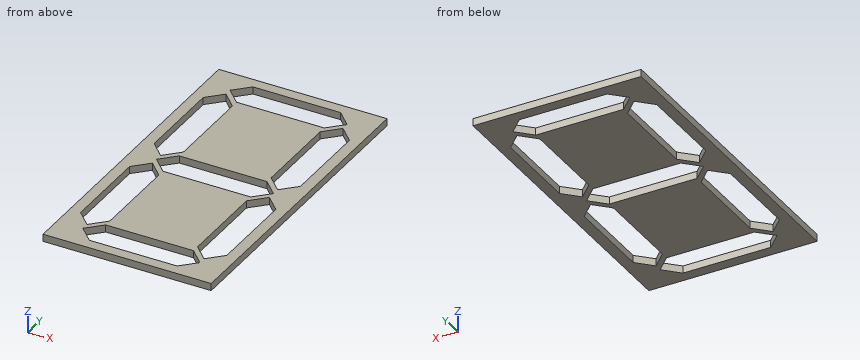
```python
from build123d import *

# Parameters (mm, degrees)
BOX011_W         = 46
BOX011_H         = 4
BOX011_DEPTH     = 10
BOX010_W         = 1
BOX010_H         = 90
BOX010_DEPTH     = 2
BOX_W            = 1
BOX_H            = 90
BOX_DEPTH        = 2
EXTRUDE006_DEPTH = 10
EXTRUDE005_DEPTH = 10
EXTRUDE004_DEPTH = 10
EXTRUDE_DEPTH    = 10
EXTRUDE003_DEPTH = 10
EXTRUDE002_DEPTH = 10
EXTRUDE001_DEPTH = 10
BOX001_W         = 44
BOX001_H         = 90
BOX001_DEPTH     = 2


with BuildPart() as cube011:
    # Box011 → Box011 (new body)
    with BuildSketch(Plane(origin=(-1, 86, -4), x_dir=(1, 0, 0), z_dir=(0, 0, 1))):
        with Locations((23, 2)):
            Rectangle(BOX011_W, BOX011_H)
    extrude(amount=BOX011_DEPTH)


with BuildPart() as cube010:
    # Box010 → Box010 (new body)
    with BuildSketch(Plane(origin=(44, 0, 0), x_dir=(1, 0, 0), z_dir=(0, 0, 1))):
        with Locations((0.5, 45)):
            Rectangle(BOX010_W, BOX010_H)
    extrude(amount=BOX010_DEPTH)


with BuildPart() as cube:
    # Box → Box (new body)
    with BuildSketch(Plane(origin=(-1, 0, 0), x_dir=(1, 0, 0), z_dir=(0, 0, 1))):
        with Locations((0.5, 45)):
            Rectangle(BOX_W, BOX_H)
    extrude(amount=BOX_DEPTH)


with BuildPart() as extrude_g:
    # Sketch008 (on Face6 of Box006) → Extrude006 (new body)
    with BuildSketch(Plane.XY.offset(10)):
        Polygon((10, 47), (6, 43), (10, 39), (34, 39), (38, 43), (34, 47), align=None)
    extrude(amount=EXTRUDE006_DEPTH)


with BuildPart() as extrude_g_1:
    # Extrude006 placement: moved
    add(extrude_g.part.moved(Location((0, 0, -14))))


with BuildPart() as extrude_f:
    # Sketch010 (on Face6 of Box008) → Extrude005 (new body)
    with BuildSketch(Plane.XY.offset(10)):
        Polygon((6, 77), (10, 73), (10, 49), (6, 45), (2, 49), (2, 73), align=None)
    extrude(amount=EXTRUDE005_DEPTH)


with BuildPart() as extrude_f_1:
    # Extrude005 placement: moved
    add(extrude_f.part.moved(Location((0, 0, -14))))


with BuildPart() as extrude_e:
    # Sketch011 (on Face6 of Box009) → Extrude004 (new body)
    with BuildSketch(Plane.XY.offset(10)):
        Polygon((6, 41), (10, 37), (10, 13), (6, 9), (2, 13), (2, 37), align=None)
    extrude(amount=EXTRUDE004_DEPTH)


with BuildPart() as extrude_e_1:
    # Extrude004 placement: moved
    add(extrude_e.part.moved(Location((0, 0, -14))))


with BuildPart() as extrude_d:
    # Sketch003 (on Face6 of Box001) → Extrude (new body)
    with BuildSketch(Plane.XY.offset(2)):
        Polygon((10, 11), (6, 7), (10, 3), (34, 3), (38, 7), (34, 11), align=None)
    extrude(amount=EXTRUDE_DEPTH)


with BuildPart() as extrude_d_1:
    # Extrude placement: moved
    add(extrude_d.part.moved(Location((0, 0, -6))))


with BuildPart() as extrude_c:
    # Sketch006 (on Face6 of Box004) → Extrude003 (new body)
    with BuildSketch(Plane.XY.offset(10)):
        Polygon((38, 41), (42, 37), (42, 13), (38, 9), (34, 13), (34, 37), align=None)
    extrude(amount=EXTRUDE003_DEPTH)


with BuildPart() as extrude_c_1:
    # Extrude003 placement: moved
    add(extrude_c.part.moved(Location((0, 0, -14))))


with BuildPart() as extrude_b:
    # Sketch007 (on Face6 of Box005) → Extrude002 (new body)
    with BuildSketch(Plane.XY.offset(10)):
        Polygon((38, 77), (42, 73), (42, 49), (38, 45), (34, 49), (34, 73), align=None)
    extrude(amount=EXTRUDE002_DEPTH)


with BuildPart() as extrude_b_1:
    # Extrude002 placement: moved
    add(extrude_b.part.moved(Location((0, 0, -14))))


with BuildPart() as extrude_a:
    # Sketch009 (on Face6 of Box007) → Extrude001 (new body)
    with BuildSketch(Plane.XY.offset(10)):
        Polygon((10, 83), (6, 79), (10, 75), (34, 75), (38, 79), (34, 83), align=None)
    extrude(amount=EXTRUDE001_DEPTH)


with BuildPart() as extrude_a_1:
    # Extrude001 placement: moved
    add(extrude_a.part.moved(Location((0, 0, -14))))


with BuildPart() as cut007:
    # Box001 → Box001 (new body)
    with BuildSketch(Plane.XY):
        with Locations((22, 45)):
            Rectangle(BOX001_W, BOX001_H)
    extrude(amount=BOX001_DEPTH)

    # Cut: cut Extrude_A
    add(extrude_a_1.part, mode=Mode.SUBTRACT)

    # Cut001: cut Extrude_B
    add(extrude_b_1.part, mode=Mode.SUBTRACT)

    # Cut002: cut Extrude_C
    add(extrude_c_1.part, mode=Mode.SUBTRACT)

    # Cut003: cut Extrude_D
    add(extrude_d_1.part, mode=Mode.SUBTRACT)

    # Cut004: cut Extrude_E
    add(extrude_e_1.part, mode=Mode.SUBTRACT)

    # Cut005: cut Extrude_F
    add(extrude_f_1.part, mode=Mode.SUBTRACT)

    # Cut006: cut Extrude_G
    add(extrude_g_1.part, mode=Mode.SUBTRACT)

    # Fusion: union Cube
    add(cube.part)

    # Fusion001: union Cube010
    add(cube010.part)

    # Cut007: cut Cube011
    add(cube011.part, mode=Mode.SUBTRACT)


solid = cut007.part
```
Read the model definition and answer for the solid it produces. Units are mm, in the model's axes. Coordinates: 2 decimals unless noted, no trailing zeros. Write each loop counter-clockwise with the first axis right and the second up, starting at its lowest first coordinate (ties: lowest second). Pieces come first, ordered by that corner, then holes. Notation, with made-up numbers: (30, 87) -> (87, 87) arc R20 cw to (87, 101) -> close; hole circle Ø8 at (56, 78). An arc over 180 degrees is marked (long way). Answer as a JSON object with one key per item and string values.
Q1. The part is cut by section C-C on x = 19. Give the vertices of the cut face in (y, z).
The answers:
{"outline": "(0, 0) -> (3, 0) -> (3, 2) -> (0, 2) -> close; (11, 0) -> (39, 0) -> (39, 2) -> (11, 2) -> close; (47, 0) -> (75, 0) -> (75, 2) -> (47, 2) -> close; (83, 0) -> (86, 0) -> (86, 2) -> (83, 2) -> close"}
Q2. The part is cut by section A-A on x = 35. Give the vertices of the cut face in (y, z).
The answers:
{"outline": "(0, 0) -> (4, 0) -> (4, 2) -> (0, 2) -> close; (10, 0) -> (12, 0) -> (12, 2) -> (10, 2) -> close; (38, 0) -> (40, 0) -> (40, 2) -> (38, 2) -> close; (46, 0) -> (48, 0) -> (48, 2) -> (46, 2) -> close; (74, 0) -> (76, 0) -> (76, 2) -> (74, 2) -> close; (82, 0) -> (86, 0) -> (86, 2) -> (82, 2) -> close"}
Q3. Consider line 1 (X direction, y = 69.5, z = 1.95); line 2 (Y direction, x = 21, z = 1.6); line 3 (Y direction, x = 8.5, z = 0.9). Determine where each line is inside the solid, lowest interval first. Write a range as [from, to].
The answers:
{"line 1": "x = [-1, 2], [10, 34], [42, 45]", "line 2": "y = [0, 3], [11, 39], [47, 75], [83, 86]", "line 3": "y = [0, 4.5], [9.5, 11.5], [38.5, 40.5], [45.5, 47.5], [74.5, 76.5], [81.5, 86]"}
Q4. The part is cut by section D-D on x = 4. Give the vertices of the cut face in (y, z).
The answers:
{"outline": "(0, 0) -> (11, 0) -> (11, 2) -> (0, 2) -> close; (39, 0) -> (47, 0) -> (47, 2) -> (39, 2) -> close; (75, 0) -> (86, 0) -> (86, 2) -> (75, 2) -> close"}
Q5. The part is cut by section B-B on y = 53. Give the vertices of the cut face in (x, z), then the cut area to 3 significant figures.
The answers:
{"outline": "(-1, 0) -> (2, 0) -> (2, 2) -> (-1, 2) -> close; (10, 0) -> (34, 0) -> (34, 2) -> (10, 2) -> close; (42, 0) -> (45, 0) -> (45, 2) -> (42, 2) -> close", "area": "60.0 mm2"}
